from build123d import *

# Parameters (mm, degrees)
F0_W     = 75
F0_H     = 12
F0_R     = 2.6
F1_DEPTH = 7.2
F2_R     = 2.6
F3_DEPTH = 5.2
F5_DEPTH = 10
F6_R     = 5


with BuildPart() as f1:
    # F0 (on Top) → F1 (new body)
    with BuildSketch(Plane.XY):
        Rectangle(F0_W, F0_H)
        with Locations((-22, 0)):
            Circle(F0_R, mode=Mode.SUBTRACT)
        Circle(F0_R, mode=Mode.SUBTRACT)
        with Locations((22, 0)):
            Circle(F0_R, mode=Mode.SUBTRACT)
    extrude(amount=F1_DEPTH)

    # F2 (on face) → F3 (cut)
    with BuildSketch(Plane.XY.offset(7.2)):
        Polygon((4, -2.309401), (4, 2.309401), (0, 4.618802), (-4, 2.309401), (-4, -2.309401), (-4, -6), (4, -6), align=None)
        Circle(F2_R, mode=Mode.SUBTRACT)
    extrude(amount=-F3_DEPTH, mode=Mode.SUBTRACT)

    # F4 (on face) → F5 (join)
    with BuildSketch(Plane.XZ.offset(6)):
        Polygon((31, 10), (-31, 10), (-37.5, 7.2), (37.5, 7.2), align=None)
    extrude(amount=-F5_DEPTH)

    # F6
    f6_edges = [f1.edges().sort_by_distance(p)[0] for p in [
        (-31, -1, 10),
        (31, -1, 10),
    ]]
    fillet(f6_edges, radius=F6_R)


solid = f1.part
Work out the finished part from the listing and answer in its coordinate system (mm). A direction names the side the tool comes from. Give positions to 0.01 mm unless a question says otherwise; leave off trailing zeros. Order: outer loops, then holes, each group sorted by start corner. A loop starts at its lowest first (then second) coordinate and runs counter-clockwise, first axis right, second up. Notation, with made-up numbers: (70.5, 16) - (105.5, 16) arc R18 cw to (105.5, 23) - close; hole circle Ø5 at (83, 18.5). An arc over 180 degrees is marked (long way). Answer as CSV lines item,"result". Start each with the question number.
Q1. Find the intervals of material crossed by L1, parallel to Y at x = 0, z = 1.5; L2, parallel to Z at x = -3.5, y = 0.5; L3, parallel to X at y = 0.5, z = 1.75, in increasing order. Write a range as [from, to].
Q2. The part is cut by section D-D (z = 4). Write down the section's boundary in (x, y), then the cut area to 3 significant figures.
Q3. The part is cut by section C-C (x = 23). Write down the section's boundary in (y, z).
Q4. For faces 1 (the face through (-1, 4, 9)), 2 (the face through (-1.97, 3.48, 4.64)), 3 (the face through (-34.685, -1.07, 8.413)), 4 (the face through (24.48, 0.78, 3.55)), determine the directions among +Z, -Z, +X, -X, +Y, -Y from which every point of the face is accessible in a straight line to the end or side of a thin tool.
Q5. The mould has two halves that part along Y. Classify faces 5 (the face through (-19.52, 0.78, 3.55)), 6 (the face through (-1, 5, 7.2)), 7 (the face through (-1, 6, 4)): +Y half, -Y half, draft (parallel to the pull), parting line (faces both ways), or undercut.
Q6. The part is cut by section A-A (z = 1). Write down the section's boundary in (x, y), then the cut area to 3 significant figures.
Q7. The part is cut by section B-B (y = -4). Write down the section's boundary in (x, z), then the cut area to 3 significant figures.
Q8. Given pin 1 Ø4 at (x, y) = (22, 0) entering from -Z; pin 2 Ø1.5 at (x, z) = (0, 5) entering from -Y; pin 3 Ø0.8 at (x, z) = (18, 9) entering from +Y, each flat-ended and moving along its own axis, determine where each tip first touches the part or whether it passes through.
Check result:
1,L1,"y = [-6, -2.6], [2.6, 6]"
1,L2,"z = [0, 2], [7.2, 10]"
1,L3,"x = [-37.5, -24.55], [-19.45, -2.55], [2.55, 19.45], [24.55, 37.5]"
2,outline,"(-37.5, -6) - (-4, -6) - (-4, 2.31) - (0, 4.62) - (4, 2.31) - (4, -6) - (37.5, -6) - (37.5, 6) - (-37.5, 6) - close; hole circle Ø5.2 at (-22, 0); hole circle Ø5.2 at (22, 0)"
2,area,"782 mm²"
3,outline,"(-6, 0) - (-2.4, 0) - (-2.4, 7.2) - (2.4, 7.2) - (2.4, 0) - (6, 0) - (6, 7.2) - (4, 7.2) - (4, 10) - (-6, 10) - close"
4,face 1,"+Z, +X, -X, +Y"
4,face 2,"-Y"
4,face 3,"+Z, -X, +Y, -Y"
4,face 4,"-Z"
5,face 5,"undercut"
5,face 6,"draft"
5,face 7,"+Y half"
6,outline,"(-37.5, -6) - (37.5, -6) - (37.5, 6) - (-37.5, 6) - close; hole circle Ø5.2 at (-22, 0); hole circle Ø5.2 at (0, 0); hole circle Ø5.2 at (22, 0)"
6,area,"836 mm²"
7,outline,"(-37.5, 0) - (37.5, 0) - (37.5, 7.2) - (31.95, 9.59) arc R5 ccw to (29.97, 10) - (-29.97, 10) arc R5 ccw to (-31.95, 9.59) - (-37.5, 7.2) - close; hole (-4, 2) - (4, 2) - (4, 7.2) - (-4, 7.2) - close"
7,area,"690 mm²"
8,pin 1,"stops at z = 7.2"
8,pin 2,"stops at y = 4.19"
8,pin 3,"stops at y = 4"
